Part model, mm, in its own coordinate system. Face numbers are marked on the shaded views. A direction names the side the tool comes from. Give positions to 0.01 mm unless a question says otherwise; leave off trailing zeros. Order: outer loops, then holes, each group sorted by start corner. A loop starts at its lowest first (then second) coordinate and runs counter-clockwise, first axis right, second up.
1. Slice it at B-B on x = 21.5. List the corners of the cut face in (y, z), and give its area (3 significant figures).
2. Drop flat-ended pins along their axis: pin 1 Ø7.5 at (x, z) = (21.5, 21.5) entering from +Y; pin 2 Ø3 at (x, z) = (11, 8) entering from -Y. Give the stop position or say it passes through.
3. Which spindle directions (+Z, -Z, +X, -X, +Y, -Y) get a long thin tool onto all of the face, cutting with end or side? Do the marked faces 1 and 2. Say none if no direction does.
4. Slice it at D-D on z = -2. List the corners of the cut face in (x, y), and give its area (3 significant figures).
5. Slice it at C-C on x = 2.5. List the corners of the cut face in (y, z), and give its area (3 significant figures).
6. Slice it at A-A on z = -21.5. List the corners of the cut face in (x, y), and give its area (3 significant figures).
7. Probe line 1 (X direction, y = 2.85, z = 21.5); line 2 (X direction, y = 1.5, z = -24); line 3 (Z direction, x = 20, y = 2.25). List the from-to ranges inside material, lowest first.
from build123d import *

# Parameters (mm, degrees)
SKETCH1_W           = 60
SKETCH1_H           = 60
BOSS_EXTRUDE1_DEPTH = 4
SKETCH2_W           = 28
SKETCH2_H           = 28
BOSS_EXTRUDE2_DEPTH = 6
DRAFT1_ANGLE        = 8
FILLET1_R           = 1
SKETCH3_R           = 2.794
CUT_EXTRUDE1_DEPTH  = 43.848570571


with BuildPart() as part:
    # Sketch1 → Boss-Extrude1 (new body)
    with BuildSketch(Plane(origin=(0, 0, 0), x_dir=(1, 0, 0), z_dir=(0, 1, 0))):
        Rectangle(SKETCH1_W, SKETCH1_H)
    extrude(amount=BOSS_EXTRUDE1_DEPTH)

    # Sketch2 → Boss-Extrude2 (add)
    with BuildSketch(Plane(origin=(0, 4, 0), x_dir=(1, 0, 0), z_dir=(0, 1, 0))):
        Rectangle(SKETCH2_W, SKETCH2_H)
    extrude(amount=BOSS_EXTRUDE2_DEPTH)

    # Draft1
    draft1_faces = [part.faces().sort_by_distance(p)[0] for p in [
        (-14, 7, 0),
        (0, 7, -14),
        (14, 7, 0),
        (0, 7, 14),
    ]]
    draft(draft1_faces, Plane.ZX.offset(10), DRAFT1_ANGLE)

    # Fillet1
    fillet1_edges = [part.edges().sort_by_distance(p)[0] for p in [
        (14.843245008, 4, 0),
        (0, 4, -14.843245008),
        (-14.843245008, 4, 0),
        (0, 4, 14.843245008),
        (14, 10, 0),
        (0, 10, -14),
        (-14, 10, 0),
        (0, 10, 14),
    ]]
    fillet(fillet1_edges, radius=FILLET1_R)

    # Sketch3 → Cut-Extrude1 (cut, through all)
    with BuildSketch(Plane(origin=(0, 4, 0), x_dir=(1, 0, 0), z_dir=(0, 1, 0))):
        with Locations(Location((-21.5, 21.5, 0), (0, 0, 270))):
            Circle(SKETCH3_R)
        with Locations(Location((21.5, 21.5, 0), (0, 0, 90))):
            Circle(SKETCH3_R)
        with Locations(Location((21.5, -21.5, 0), (0, 0, 270))):
            Circle(SKETCH3_R)
        with Locations(Location((-21.5, -21.5, 0), (0, 0, 90))):
            Circle(SKETCH3_R)
    extrude(amount=-CUT_EXTRUDE1_DEPTH, mode=Mode.SUBTRACT)


solid = part.part
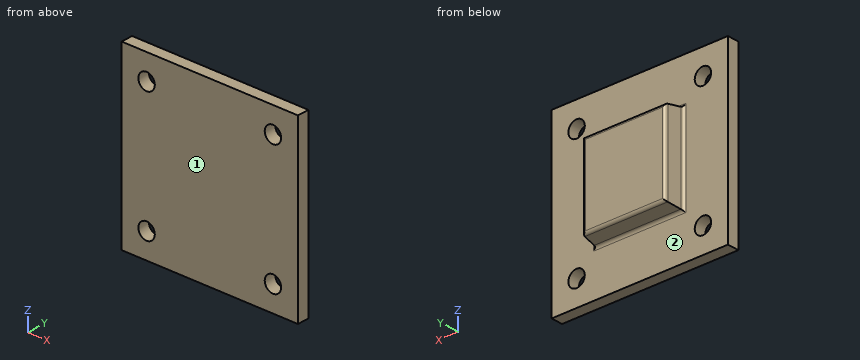
Data:
1. outline: (0, -30) - (4, -30) - (4, -24.29) - (0, -24.29) - close; (0, -18.71) - (4, -18.71) - (4, 18.71) - (0, 18.71) - close; (0, 24.29) - (4, 24.29) - (4, 30) - (0, 30) - close
1. area: 195 mm2
2. pin 1: stops at y = 4
2. pin 2: stops at y = 0
3. face 1: +Z, -Z, +X, -X, -Y
3. face 2: +Y
4. outline: (-30, 0) - (30, 0) - (30, 4) - (15.71, 4) arc R1 cw to (14.72, 4.86) - (14.12, 9.14) arc R1 ccw to (13.13, 10) - (-13.13, 10) arc R1 ccw to (-14.12, 9.14) - (-14.72, 4.86) arc R1 cw to (-15.71, 4) - (-30, 4) - close
4. area: 413 mm2
5. outline: (0, -30) - (4, -30) - (4, -15.71) arc R1 cw to (4.86, -14.72) - (9.14, -14.12) arc R1 ccw to (10, -13.13) - (10, 13.13) arc R1 ccw to (9.14, 14.12) - (4.86, 14.72) arc R1 cw to (4, 15.71) - (4, 30) - (0, 30) - close
5. area: 413 mm2
6. outline: (-30, 0) - (-24.29, 0) - (-24.29, 4) - (-30, 4) - close; (-18.71, 0) - (18.71, 0) - (18.71, 4) - (-18.71, 4) - close; (24.29, 0) - (30, 0) - (30, 4) - (24.29, 4) - close
6. area: 195 mm2
7. line 1: x = -30 to -24.29, -18.71 to 18.71, 24.29 to 30
7. line 2: x = -30 to -22.75, -20.25 to 20.25, 22.75 to 30
7. line 3: z = -30 to -23.86, -19.14 to 19.14, 23.86 to 30
